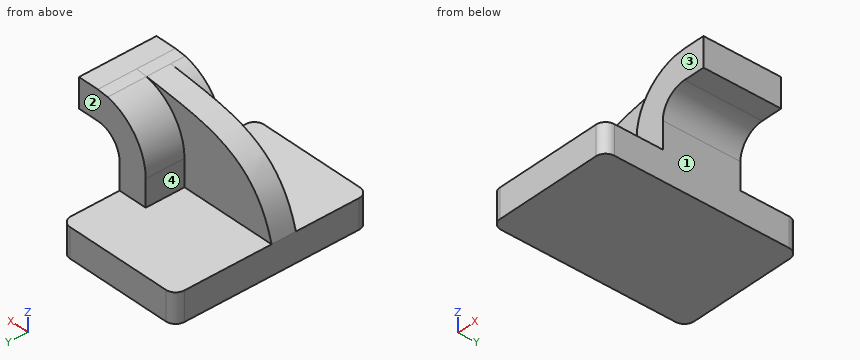
from build123d import *

# Parameters (mm, degrees)
F1_DEPTH = 63.5
F0_W     = 10.6006153176
F0_H     = 19.05
F2_DEPTH = 25.4
F3_DEPTH = 15.875
F4_R     = 6.35


with BuildPart() as f1:
    # F0 (on Front) → F1 (new body, symmetric)
    with BuildSketch(Plane.XZ):
        Polygon((22.225, 9.525), (-41.275, 9.525), (-41.275, -9.525), (41.275, -9.525), (41.275, 9.525), align=None)
    extrude(amount=F1_DEPTH, both=True)

    # F0 (on Front) → F2 (join, symmetric)
    with BuildSketch(Plane.XZ):
        with BuildLine():
            Line((22.225, 27.0002), (22.225, 9.525))
            Line((22.225, 9.525), (41.275, 9.525))
            Line((41.275, 9.525), (41.275, 27.0002))
            ThreePointArc((41.275, 27.0002), (45.9246798487, 38.2255201513), (57.15, 42.8752))
            Line((57.15, 42.8752), (60.325, 42.8752))
            Line((60.325, 42.8752), (60.325, 61.9252))
            Line((60.325, 61.9252), (57.15, 61.9252))
            add(Edge.make_bspline(
                [(49.9755002141, 61.180343034), (52.3379879204, 61.4198350187), (54.7300422112, 61.6659292139), (57.15, 61.9252)],
                knots=[105.9316998893, 105.9316998893, 105.9316998893, 105.9316998893, 111.5045361635, 111.5045361635, 111.5045361635, 111.5045361635], degree=3))
            ThreePointArc((49.9755002141, 61.180343034), (30.036119514, 49.0136756454), (22.225, 27.0002))
        make_face()
        with Locations((65.6253076588, 52.4002)):
            Rectangle(F0_W, F0_H)
    extrude(amount=F2_DEPTH, both=True)

    # F0 (on Front) → F3 (join)
    with BuildSketch(Plane.XZ):
        with BuildLine():
            add(Edge.make_bspline(
                [(-41.275, 9.525), (-29.1563910851, 54.461089134), (5.067965455, 56.6279406654), (49.9755002141, 61.180343034)],
                knots=[0, 0, 0, 0, 105.9316998893, 105.9316998893, 105.9316998893, 105.9316998893], degree=3))
            Line((-41.275, 9.525), (22.225, 9.525))
            Line((22.225, 9.525), (22.225, 27.0002))
            ThreePointArc((22.225, 27.0002), (30.036119514, 49.0136756454), (49.9755002141, 61.180343034))
        make_face()
    extrude(amount=F3_DEPTH)

    # F4
    f4_edges = [f1.edges().sort_by_distance(p)[0] for p in [
        (-41.275, -63.5, 0),
        (41.275, -63.5, 0),
        (-41.275, 63.5, 0),
        (41.275, 63.5, 0),
    ]]
    fillet(f4_edges, radius=F4_R)


solid = f1.part
Work out the finished part from the listing and answer in its coordinate system (mm). Face numbers are marked on the shaded views. A direction names the side the tool comes from. Coordinates: 2 decimals unless noted, no trailing zeros. Write each loop counter-clockwise with the first axis right and the second up, starting at its lowest first coordinate (ties: lowest second). Pieces come first, ordered by that corner, then holes. Notation, with made-up numbers: (26, 4) - (58, 4) arc R14 ccw to (58, 27) - close; hole circle Ø6 at (-22, 49.25). An arc over 180 degrees is marked (long way). One line per question, with ' | ' between items.
1) Flat-ended cylindrical pins translate along their axes: P1, Ø12, axis at y = -43, z = 5.5, coming from the +X side (3 decimals); P2, Ø4, axis at x = 14, z = 30, coming from the -Y side (3 decimals); P3, Ø24.5, axis at x = 43.5, z = 25.5, coming from the -Y side. Find the tip coordinate at first contact, or state that the pin passes through.
Checks:
P1: x = 41.275 | P2: y = -15.875 | P3: y = -25.4
2) Find section A-A, the plane z = -3.5. Determine the outline of the cut face in (x, y) (3 decimals).
Checks:
outline: (-41.275, -57.15) arc R6.35 ccw to (-34.925, -63.5) - (34.925, -63.5) arc R6.35 ccw to (41.275, -57.15) - (41.275, 57.15) arc R6.35 ccw to (34.925, 63.5) - (-34.925, 63.5) arc R6.35 ccw to (-41.275, 57.15) - close
3) Find section B-B, the plane y = -32. Determine the outline of the cut face in (x, z) (3 decimals).
Checks:
outline: (-41.275, -9.525) - (41.275, -9.525) - (41.275, 9.525) - (-41.275, 9.525) - close
4) For the marked faces 1, 2, 3 and 4, determine the directions among +Z, -Z, +X, -X, +Y, -Y from which every point of the face is accessible in a straight line to the end or side of a thin tool.
Checks:
face 1: -Z, +X, +Y, -Y | face 2: +Z, +X, -X, +Y | face 3: +Z, +X, -X, -Y | face 4: +Z, -X, +Y
5) Consider probe 1 along Z at (x, y) = (-28.5, -55) (3 decimals); probe 2 along Y at (x, z) = (11, 36.5) (3 decimals); probe 3 along X at (y, z) = (-19, 1.5) (3 decimals). Determine where each line is inside the solid, lowest interval first. Write a range as [from, to].
Checks:
probe 1: [-9.525, 9.525] | probe 2: [-15.875, 0] | probe 3: [-41.275, 41.275]
